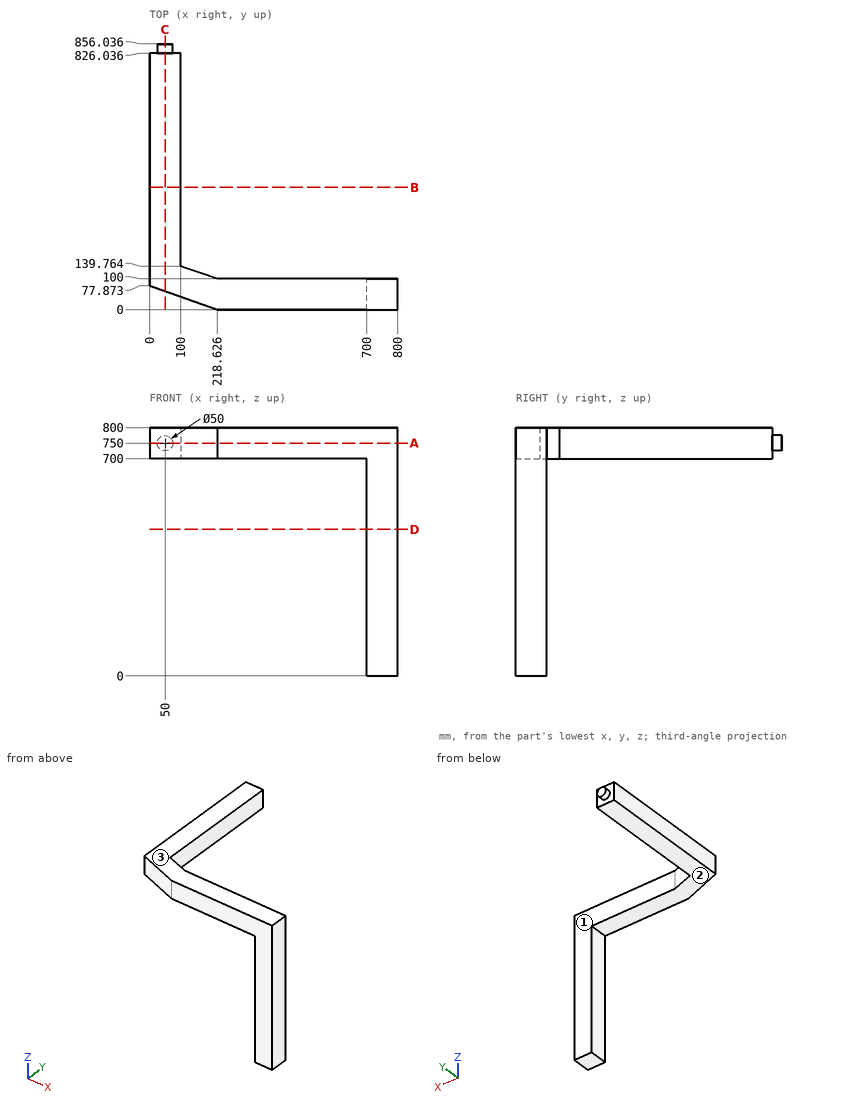
Here's the drawing with two shaded views (mm, measured from the low corner). I have some questions. A direction names the side the tool comes from. Round coordinates to 2 decimals unless told otherwise and drop trailing zeros. Loops run counter-clockwise (first coordinate to the right, second up) from the corner with the lowest first, then second, coordinate; pieces in that order, holes last. Notation, with made-up numbers: M 19,50.5 L 51,50.5 A27 ccw 51,71.5 Z; hole C 1,82 d11. An arc over 180 degrees is marked long. Answer as CSV lines item,"result".
1) Imagine slicing it at C-C on x = 50. List the corners of the cut face in (y, z) for me (1 decimal), and give its area (3 significant figures).
From the geometry:
outline,"M 60.1,700 L 826,700 L 826,725 L 856,725 L 856,775 L 826,775 L 826,800 L 60.1,800 Z"
area,"78,100 mm^2"
2) Imagine slicing it at D-D on z = 472.5. List the corners of the cut face in (x, y) for me, and give its area (3 significant figures).
From the geometry:
outline,"M 700,0 L 800,0 L 800,100 L 700,100 Z"
area,"10,000 mm^2"
3) Which directions (+Z, -Z, +X, -X, +Y, -Y) give clear straight access to the entire face, cutting with the end or side of a thin tool? Please do the marked faces 1, 2 and 3.
From the geometry:
face 1,"+Z, -Z, +X, +Y"
face 2,"-Z, -X, +Y, -Y"
face 3,"+Z, +X, -X, +Y, -Y"
4) If I drill on probe 1 along X at (y, z) = (45, 669.5); probe 2 along X at (y, z) = (787, 727), over which ranges is the centre line in solid material (lowest first)?
From the geometry:
probe 1,"700 to 800"
probe 2,"0 to 100"
5) Imagine slicing it at A-A on z = 750. List the corners of the cut face in (x, y) for me (1 decimal), and give its area (3 significant figures).
From the geometry:
outline,"M 0,77.9 L 218.6,0 L 800,0 L 800,100 L 218.6,100 L 100,139.8 L 100,826 L 75,826 L 75,856 L 25,856 L 25,826 L 0,826 Z"
area,"148,000 mm^2"
6) Imagine slicing it at B-B on y = 394. List the corners of the cut face in (x, z) for me.
From the geometry:
outline,"M 0,700 L 100,700 L 100,800 L 0,800 Z"
